Here's how the part is built. I have some questions about the finished solid (model axes, mm). A direction names the side the tool comes from. Coordinates: 2 decimals unless noted, no trailing zeros. Write each loop counter-clockwise with the first axis right and the second up, starting at its lowest first coordinate (ties: lowest second). Pieces come first, ordered by that corner, then holes.
Item 1: If we section it at C-C (y = 64): Please give me the cut outline in (x, z) (3 decimals).
Item 2: For faces 5 (the face through (20, 19, 3.375)), 6 (the face through (23.08, 58.08, -2.46)), 7 (the face through (40, 51, 22)), which set-ups out of +Z, -Z, +X, -X, +Y, -Y let a thin tool reach every point of the face, with its end or its side?
Item 3: If we section it at B-B (x = 20): Please give me the cut outline in (y, z) (3 decimals).
Item 4: We'd pull the mould along Y, two halves only. Please class faces 1 (the face through (8.124, 15.594, 1.711)), 2 (the face through (20, 43, 0)), 3 (the face through (20, 85, 22)), 4 (the face through (18.12, 66.95, 20.35)): +Y half, -Y half, draft (parallel to the pull), parting line (faces both ways), or undercut.
Item 5: If we section it at A-A (y = 19.2): Please give me the cut outline in (x, z) (3 decimals), then the cut area to 3 significant figures.
Item 6: If we section it at D-D (x = 30): Please give me the cut outline in (y, z) (3 decimals), then the cut area to 3 significant figures.
Item 7: If I drill on line 1 (X direction, y = 19, z = 1); line 2 (Y direction, x = 20, z = 16); line 3 (Y direction, x = 30, z = 2.1) (3 decimals), over which ranges is the centre line in solid material (lowest first)?
Item 8: I'm going to push a flat-ended pin straight in: pin 1 Ø10.5 at (x, y) = (10, 19.2) entering from -Z. Where does the tip first touch, or does it pass through?
from build123d import *

# Parameters (mm, degrees)
ESQUISSE1_W                  = 40
ESQUISSE1_H                  = 85
BOSS_EXTRU_1_DEPTH           = 45
ESQUISSE2_W                  = 38.25
ESQUISSE2_H                  = 38.25
ENL_V_MAT_EXTRU_1_DEPTH      = 105.16333328
ENL_V_MAT_EXTRU_2_DEPTH      = 103.75038017
ENL_V_MAT_EXTRU_2_DEPTH_BACK = 103.75038017
ESQUISSE3_R                  = 4.065
ESQUISSE6_R                  = 6.675
BOSS_EXTRU_2_DEPTH           = 5
ENL_V_MAT_EXTRU_4_DEPTH      = 105.16333328
ENL_V_MAT_EXTRU_4_DEPTH_BACK = 105.16333328
ESQUISSE4_R                  = 3.5


with BuildPart() as part:
    # Esquisse1 → Boss.-Extru.1 (new body)
    with BuildSketch(Plane.XY):
        with Locations((20, 42.5)):
            Rectangle(ESQUISSE1_W, ESQUISSE1_H)
    extrude(amount=BOSS_EXTRU_1_DEPTH)

    # Esquisse2 → Enlèv. mat.-Extru.1 (cut, through all)
    with BuildSketch(Plane(origin=(40, 0, 0), x_dir=(0, 0, -1), z_dir=(1, 0, 0))):
        with Locations((-22.5, 19.125)):
            Rectangle(ESQUISSE2_W, ESQUISSE2_H)
    extrude(amount=-ENL_V_MAT_EXTRU_1_DEPTH, mode=Mode.SUBTRACT)

    # Esquisse3 → Enlèv. mat.-Extru.2 (cut, two sides: drawn at the far end of the back side and taken through both)
    with BuildSketch(Plane(origin=(0, 0, 41.625), x_dir=(-1, 0, 0), z_dir=(0, 0, -1)).offset(-ENL_V_MAT_EXTRU_2_DEPTH_BACK)):
        with Locations((-30, 19.2)):
            Circle(ESQUISSE3_R)
        with Locations((-10, 19.2)):
            Circle(ESQUISSE3_R)
    extrude(amount=ENL_V_MAT_EXTRU_2_DEPTH + ENL_V_MAT_EXTRU_2_DEPTH_BACK, mode=Mode.SUBTRACT)

    # Esquisse6 → Boss.-Extru.2 (add)
    with BuildSketch(Plane.XY):
        with Locations((20, 64)):
            Circle(ESQUISSE6_R)
    extrude(amount=-BOSS_EXTRU_2_DEPTH)

    # Esquisse4 → Enlèv. mat.-Extru.4 (cut, two sides: drawn at the far end of the back side and taken through both)
    with BuildSketch(Plane(origin=(0, 0, 0), x_dir=(-1, 0, 0), z_dir=(0, 0, -1)).offset(-ENL_V_MAT_EXTRU_4_DEPTH_BACK)):
        with Locations((-20, 64)):
            Circle(ESQUISSE4_R)
    extrude(amount=ENL_V_MAT_EXTRU_4_DEPTH + ENL_V_MAT_EXTRU_4_DEPTH_BACK, mode=Mode.SUBTRACT)


solid = part.part
Answer list:
1. outline: (0, 0) - (13.325, 0) - (13.325, -5) - (16.5, -5) - (16.5, 45) - (0, 45) - close; (23.5, -5) - (26.675, -5) - (26.675, 0) - (40, 0) - (40, 45) - (23.5, 45) - close
2. face 5: +X, -X, -Y
2. face 6: -Z
2. face 7: +Z, -Z, +X, +Y, -Y
3. outline: (0, 0) - (57.325, 0) - (57.325, -5) - (60.5, -5) - (60.5, 45) - (0, 45) - (0, 41.625) - (38.25, 41.625) - (38.25, 3.375) - (0, 3.375) - close; (67.5, -5) - (70.675, -5) - (70.675, 0) - (85, 0) - (85, 45) - (67.5, 45) - close
4. face 1: undercut
4. face 2: draft
4. face 3: +Y half
4. face 4: undercut
5. outline: (0, 0) - (5.935, 0) - (5.935, 3.375) - (0, 3.375) - close; (0, 41.625) - (5.935, 41.625) - (5.935, 45) - (0, 45) - close; (14.065, 0) - (25.935, 0) - (25.935, 3.375) - (14.065, 3.375) - close; (14.065, 41.625) - (25.935, 41.625) - (25.935, 45) - (14.065, 45) - close; (34.065, 0) - (40, 0) - (40, 3.375) - (34.065, 3.375) - close; (34.065, 41.625) - (40, 41.625) - (40, 45) - (34.065, 45) - close
5. area: 160 mm2
6. outline: (0, 0) - (15.135, 0) - (15.135, 3.375) - (0, 3.375) - close; (0, 41.625) - (15.135, 41.625) - (15.135, 45) - (0, 45) - close; (23.265, 0) - (85, 0) - (85, 45) - (23.265, 45) - (23.265, 41.625) - (38.25, 41.625) - (38.25, 3.375) - (23.265, 3.375) - close
6. area: 2,310 mm2
7. line 1: x = 0 to 5.94, 14.06 to 25.94, 34.06 to 40
7. line 2: y = 38.25 to 60.5, 67.5 to 85
7. line 3: y = 0 to 15.135, 23.265 to 85
8. pin 1: stops at z = 0
